```python
from build123d import *

# Parameters (mm, degrees)
BOSS_EXTRUDE1_DEPTH = 1.5


with BuildPart() as part:
    # Sketch1 → Revolve1 (revolve)
    with BuildSketch(Plane.XY, mode=Mode.PRIVATE) as revolve1_sk:
        Polygon((0, 0), (14.5, 0), (14.5, 3), (15.5, 3), (15.5, 4.5), (15, 4.5), (14.5, 7.5), (0, 7.5), align=None)
    revolve(revolve1_sk.sketch.rotate(Axis((0, 7.5, 0), (0, -1, 0)), 90), axis=Axis((0, 7.5, 0), (0, -1, 0)))

    # Sketch2 → Boss-Extrude1 (add)
    with BuildSketch(Plane(origin=(0, 4.5, 0), x_dir=(1, 0, 0), z_dir=(0, 1, 0))):
        with BuildLine():
            ThreePointArc((8.080445146, 12.6375), (0, 18.5), (-8.080445146, 12.6375))
            ThreePointArc((-8.080445146, 12.6375), (0, 15), (8.080445146, 12.6375))
        make_face()
    extrude(amount=-BOSS_EXTRUDE1_DEPTH)


solid = part.part
```
Model file for the job. Use its own axes, mm. A direction names the side the tool comes from. Coordinates: 2 decimals unless noted, no trailing zeros. Loops run counter-clockwise (first coordinate to the right, second up) from the corner with the lowest first, then second, coordinate; pieces in that order, holes last. Notation, with made-up numbers: (17.5, 7.25) - (25.5, 7.25) arc R21 ccw to (25.5, 13.25) - close; hole circle Ø5 at (8.5, 42.5). An arc over 180 degrees is marked (long way). Write item = value, one per line. Start each with the question number.
Item 1: Wall check: probe 1 along X at (y, z) = (5.5, -1); probe 2 along Z at (x, y) = (12.5, 2); probe 3 along Z at (x, y) = (7, 4.25). Give the ranges that are in metal, low to high. Write a range as [from, to].
Item 2: Saw through at B-B, the plane x = 0. List the corners of the cut face in (y, z).
Item 3: Saw through at C-C, the plane y = 1. List the corners of the cut face in (x, z).
Item 4: Saw through at A-A, the plane z = 0. List the corners of the cut face in (x, y), then the cut area to 3 significant figures.
Item 5: Drop flat-ended pins along their axis: pin 1 Ø5 at (x, z) = (-5, 3.5) entering from -Y; pin 2 Ø1.5 at (x, y) = (9, 5.5) entering from +Z; pin 3 Ø4 at (x, y) = (5.5, 2.5) entering from +Z. Give the stop position or say it passes through.
Item 6: 3-axis set-ups, long thin cutter, end or side, ignore diameter. For faces 1 (the face through (12.864, 1.521, 6.691)), 2 (the face through (-0.1, 4.5, -15.4)), 3 (the face through (0.57, 3.76, 15.49)): which of +Z, -Z, +X, -X, +Y, -Y reach the whole face in a straight line?
Answers:
q1.probe_1 = [-14.8, 14.8]
q1.probe_2 = [-7.35, 7.35]
q1.probe_3 = [-14.82, 13.83]
q2.outline = (0, -14.5) - (3, -14.5) - (3, -18.5) - (4.5, -18.5) - (4.5, -15) - (7.5, -14.5) - (7.5, 14.5) - (4.5, 15) - (4.5, 15.5) - (3, 15.5) - (3, 14.5) - (0, 14.5) - close
q3.outline = circle Ø29 at (0, 0)
q4.outline = (-15.5, 3) - (-14.5, 3) - (-14.5, 0) - (14.5, 0) - (14.5, 3) - (15.5, 3) - (15.5, 4.5) - (15, 4.5) - (14.5, 7.5) - (-14.5, 7.5) - (-15, 4.5) - (-15.5, 4.5) - close
q4.area = 222 mm2
q5.pin_1 = 0
q5.pin_2 = 12.35
q5.pin_3 = 15.08
q6.face_1 = -Y
q6.face_2 = +Y
q6.face_3 = +Y, -Y
